```python
from build123d import *

# Parameters (mm, degrees)
SKETCH1_R           = 2.1
BOSS_EXTRUDE1_DEPTH = 3
FILLET1_R           = 2
SKETCH3_R           = 0.8
CUT_EXTRUDE1_DEPTH  = 145.25324953
BOSS_EXTRUDE2_START = -3
BOSS_EXTRUDE2_DEPTH = 3
CUT_EXTRUDE2_DEPTH  = 145.25324953
FILLET2_R           = 2
FILLET3_R           = 10


with BuildPart() as part:
    # Sketch1 → Boss-Extrude1 (new body)
    with BuildSketch(Plane.XY):
        Polygon((-100, -80), (-100, -10), (0, -10), (0, 10), (-100, 10), (-100, 80), (-120, 80), (-120, -80), align=None)
        with Locations((-110, 70)):
            Circle(SKETCH1_R, mode=Mode.SUBTRACT)
        with Locations((-110, 50)):
            Circle(SKETCH1_R, mode=Mode.SUBTRACT)
        with Locations((-110, 30)):
            Circle(SKETCH1_R, mode=Mode.SUBTRACT)
        with Locations((-110, 10)):
            Circle(SKETCH1_R, mode=Mode.SUBTRACT)
        with Locations((-110, -10)):
            Circle(SKETCH1_R, mode=Mode.SUBTRACT)
        with Locations((-110, -30)):
            Circle(SKETCH1_R, mode=Mode.SUBTRACT)
        with Locations((-110, -50)):
            Circle(SKETCH1_R, mode=Mode.SUBTRACT)
        with Locations((-110, -70)):
            Circle(SKETCH1_R, mode=Mode.SUBTRACT)
        with Locations((-10, 0)):
            Circle(SKETCH1_R, mode=Mode.SUBTRACT)
        with Locations((-30, 0)):
            Circle(SKETCH1_R, mode=Mode.SUBTRACT)
        with Locations((-50, 0)):
            Circle(SKETCH1_R, mode=Mode.SUBTRACT)
        with Locations((-70, 0)):
            Circle(SKETCH1_R, mode=Mode.SUBTRACT)
        with Locations((-90, 0)):
            Circle(SKETCH1_R, mode=Mode.SUBTRACT)
    extrude(amount=BOSS_EXTRUDE1_DEPTH)

    # Fillet1
    fillet1_edges = [part.edges().sort_by_distance(p)[0] for p in [
        (-120, -80, 1.5),
        (-120, 80, 1.5),
        (-100, 80, 1.5),
        (0, 10, 1.5),
        (0, -10, 1.5),
        (-100, -80, 1.5),
    ]]
    fillet(fillet1_edges, radius=FILLET1_R)

    # Sketch3 → Cut-Extrude1 (cut, through all)
    with BuildSketch(Plane.XY.offset(3)):
        with Locations((-100, 10)):
            Circle(SKETCH3_R)
        with Locations((-100, -10)):
            Circle(SKETCH3_R)
    extrude(amount=-CUT_EXTRUDE1_DEPTH, mode=Mode.SUBTRACT)

    # Sketch4 → Boss-Extrude2 (add)
    with BuildSketch(Plane(origin=(0, 0, 0), x_dir=(-1, 0, 0), z_dir=(0, 0, -1)).offset(BOSS_EXTRUDE2_START)):
        with BuildLine():
            Line((0, -8), (0, -10))
            Line((0, -10), (100, -80))
            Line((100, -80), (102, -80))
            ThreePointArc((102, -80), (100.585786438, -79.414213562), (100, -78))
            Line((100, -78), (100, -10.8))
            ThreePointArc((100, -10.8), (100.565685425, -9.434314575), (99.2, -10))
            Line((99.2, -10), (2, -10))
            ThreePointArc((2, -10), (0.585786438, -9.414213562), (0, -8))
        make_face()
    extrude(amount=BOSS_EXTRUDE2_DEPTH)

    # Sketch5 → Cut-Extrude2 (cut, through all)
    with BuildSketch(Plane(origin=(0, 0, 0), x_dir=(-1, 0, 0), z_dir=(0, 0, -1))):
        Polygon((40.442619177, -20), (90, -20), (90, -54.690166576), align=None)
    extrude(amount=-CUT_EXTRUDE2_DEPTH, mode=Mode.SUBTRACT)

    # Fillet2
    fillet2_edges = [part.edges().sort_by_distance(p)[0] for p in [
        (-90, -54.690166576, 1.5),
        (-40.442619177, -20, 1.5),
        (-90, -20, 1.5),
    ]]
    fillet(fillet2_edges, radius=FILLET2_R)

    # Fillet3
    fillet3_edges = [part.edges().sort_by_distance(p)[0] for p in [
        (-100, -80, 1.5),
        (0, -10, 1.5),
    ]]
    fillet(fillet3_edges, radius=FILLET3_R)


solid = part.part
```
Here's how the part is built. I have some questions about the finished solid (model axes, mm). A direction names the side the tool comes from. Coordinates: 2 decimals unless noted, no trailing zeros. Order: outer loops, then holes, each group sorted by start corner. A loop starts at its lowest first (then second) coordinate and runs counter-clockwise, first axis right, second up. Notation, with made-up numbers: M 78.5,26.25 L 123.5,26.25 A27 cw 123.5,59.25 Z; hole C -11.5,-16.5 d7. An arc over 180 degrees is marked long. Answer as a JSON object with one key per item and string values. Group by question number.
(1) If we mould it in two halves opening along X, with no side actions, what happens to faces 3 (the face through (-1.16, -9.47, 1.48)), 4 (the face through (-110.46, -72.05, 1.48)), 5 (the face through (-72, -17, 0))? For each: released by +X, released by -X, zero draft, split by the parting line, or undercut.
(2) Suppose I cut it at C-C, the plane z = 0.65. State how many separate pieces and enclosed holes the cut face has, then the cut area to 3 significant figures.
(3) For pin 1 (4 mm diameter, centred on x = -90, y = 0, fed in from -Z); pin 2 (1 mm diameter, centred on y = 60.5, z = 2.5, fed in from +X); pin 3 (0.9 mm diameter, centred on x = -28, z = 2, fed in from +Y), each with a flat end and sliding along its axis, tell me the tip position at first contact or that it passes through.
(4) I need wall thicknesses on probe 1 along Y at (x, z) = (-50, 0.9); probe 2 along Y at (x, z) = (-10, 0.8); probe 3 along Y at (x, z) = (-54.5, 1.85). Which ranges of each line are inside material? Lowest first, please.
(5) Suppose I cut it at A-A, the plane x = -10. Please give me the cut outline in (y, z), then the cut area to 3 significant figures.
(6) Suppose I cut it at B-B, the plane y = 70. Please give me the cut outline in (x, z), then the cut area to 3 significant figures.
(7) Which directions (+Z, -Z, +X, -X, +Y, -Y) give clear straight access to the entire face, cutting with the end or side of a thin tool? Please do faces 1 (the face through (-72, -17, 3)), 2 (the face through (-66.535, -38.265, 1.479)).
Values found:
{
 "1": {"face 3": "released by +X", "face 4": "undercut", "face 5": "zero draft"},
 "2": {"separate pieces": "1", "enclosed holes": "14", "area": "7,660 mm^2"},
 "3": {"pin 1": "passes through", "pin 2": "stops at x = -100", "pin 3": "stops at y = 10"},
 "4": {"probe 1": "y = -45 to -26.69, -20 to -2.1, 2.1 to 10", "probe 2": "y = -17 to -2.1, 2.1 to 10", "probe 3": "y = -48.15 to -29.84, -20 to 10"},
 "5": {"outline": "M -17,0 L -2.1,0 L -2.1,3 L -17,3 Z; M 2.1,0 L 10,0 L 10,3 L 2.1,3 Z", "area": "68.4 mm^2"},
 "6": {"outline": "M -120,0 L -112.1,0 L -112.1,3 L -120,3 Z; M -107.9,0 L -100,0 L -100,3 L -107.9,3 Z", "area": "47.4 mm^2"},
 "7": {"face 1": "+Z, +X, -X, +Y, -Y", "face 2": "+Z, -Z"}
}
